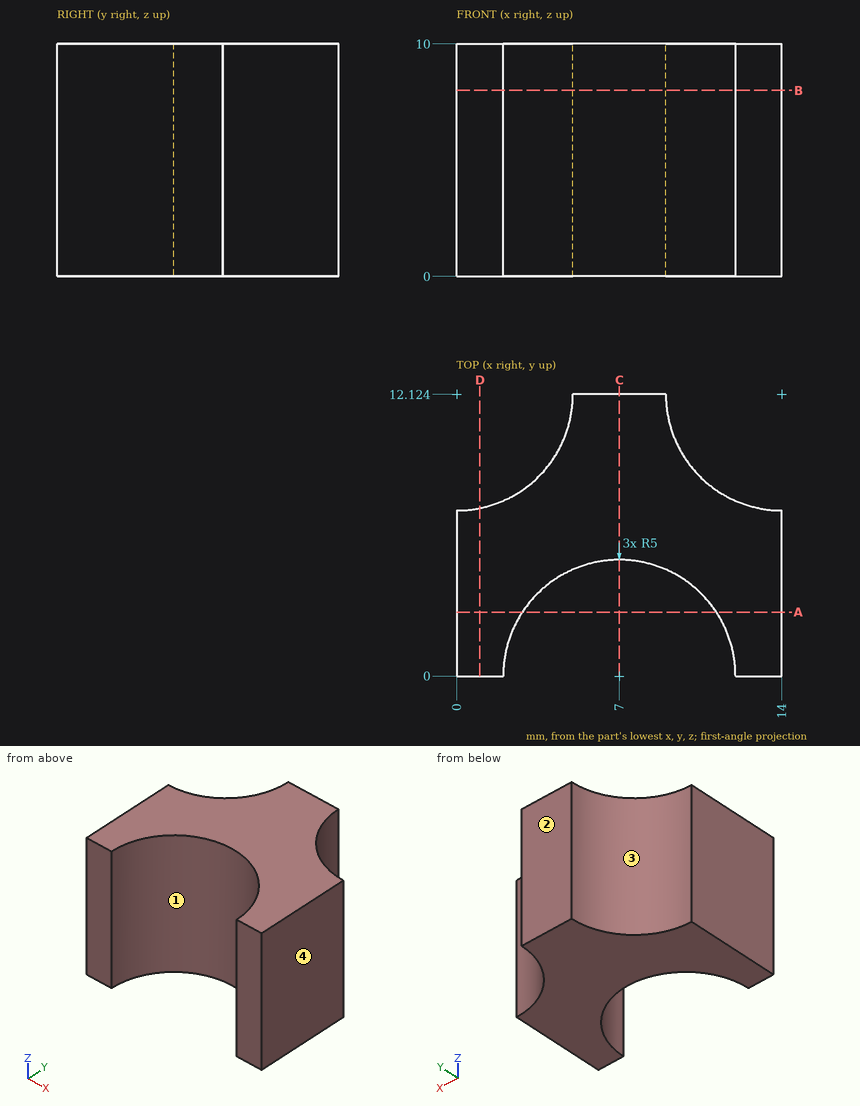
Drawing for the job (mm, zero at the part's lowest x, y, z). Give positions to 0.01 mm unless a question says otherwise; leave off trailing zeros. Write each loop counter-clockwise with the first axis right and the second up, starting at its lowest first coordinate (ties: lowest second). Pieces come first, ordered by that corner, then holes. Notation, with made-up numbers: M 40,66 L 87,66 A19 ccw 87,101 Z; hole C -33.75,-19.75 d3. An arc over 180 degrees is marked long. Return JSON: item names as keys, results as strings. Group by question number.
(1) Band-saw the part on A-A (y = 2.75). Give the cut face in (x, z).
(2) Mould opens along X. For the marked faces 1, 2, 3 and 4 say: pulls with the +X half, pulls with the -X half, needs draft (parallel to the pull), parting line crosses it, or undercut.
(3) Flat gauge pins, fed straight in: pin 1 Ø3 at (x, z) = (2.5, 8.5) entering from +Y (1 decimal); pin 2 Ø2 at (x, z) = (10, 3.5) entering from -Y. Where does each tip first touch, or does it go through?
(4) Drill centre lines: L1, parallel to X at y = 2.25, z = 1 (1 decimal); L2, parallel to X at y = 2.75, z = 4.5 (1 decimal); L3, parallel to Y at x = 8, z = 6.75 (1 decimal). Where is each one in solid material? Low to high. Write a range as [from, to].
(5) Band-saw the part on B-B (z = 8). Give the cut face in (x, y) (1 decimal).
(6) Band-saw the part on C-C (x = 7). Give the cut face in (y, z) (1 decimal).
(7) Band-saw the part on D-D (x = 1). Give the cut face in (y, z) (1 decimal).
Entries:
{
 "1": {"outline": "M 0,0 L 2.82,0 L 2.82,10 L 0,10 Z; M 11.18,0 L 14,0 L 14,10 L 11.18,10 Z"},
 "2": {"face 1": "undercut", "face 2": "needs draft", "face 3": "pulls with the -X half", "face 4": "pulls with the +X half"},
 "3": {"pin 1": "stops at y = 9.1", "pin 2": "stops at y = 3"},
 "4": {"L1": "x = [0, 2.5], [11.5, 14]", "L2": "x = [0, 2.8], [11.2, 14]", "L3": "y = [4.9, 12.1]"},
 "5": {"outline": "M 0,0 L 2,0 A5 cw 12,0 L 14,0 L 14,7.1 A5 cw 9,12.1 L 5,12.1 A5 cw 0,7.1 Z"},
 "6": {"outline": "M 5,0 L 12.1,0 L 12.1,10 L 5,10 Z"},
 "7": {"outline": "M 0,0 L 7.2,0 L 7.2,10 L 0,10 Z"}
}
